```python
from build123d import *

# Parameters (mm, degrees)
SKETCH1_R           = 8.5
SKETCH1_R_2         = 2.5
BOSS_EXTRUDE2_DEPTH = 4.5


with BuildPart() as part:
    # Sketch1 → Boss-Extrude2 (new body)
    # profile 1 of 3: a face of its own
    with BuildSketch(Plane(origin=(0, 0, 0), x_dir=(1, 0, 0), z_dir=(0, 1, 0))):
        with BuildLine():
            Line((0, 8.5), (-120, 8.5))
            ThreePointArc((-120, 8.5), (-113.98959236, 6.01040764), (-111.5, 0))
            ThreePointArc((-111.5, 0), (-113.98959236, -6.01040764), (-120, -8.5))
            Line((-120, -8.5), (0, -8.5))
            ThreePointArc((0, -8.5), (-8.5, 0), (0, 8.5))
        make_face()
    # profile 2 of 3: a face of its own
    with BuildSketch(Plane(origin=(0, 0, 0), x_dir=(1, 0, 0), z_dir=(0, 1, 0))):
        with Locations((-120, 0)):
            Circle(SKETCH1_R)
        with Locations(Location((-120, 0, 0), (0, 0, 270))):
            Circle(SKETCH1_R_2, mode=Mode.SUBTRACT)
    # profile 3 of 3: a face of its own
    with BuildSketch(Plane(origin=(0, 0, 0), x_dir=(1, 0, 0), z_dir=(0, 1, 0))):
        Circle(SKETCH1_R)
        with Locations(Location((0, 0, 0), (0, 0, 270))):
            Circle(SKETCH1_R_2, mode=Mode.SUBTRACT)
    extrude(amount=BOSS_EXTRUDE2_DEPTH)


solid = part.part
```
Part model, mm, in its own coordinate system. Give positions to 0.01 mm unless a question says otherwise; leave off trailing zeros. Order: outer loops, then holes, each group sorted by start corner. A loop starts at its lowest first (then second) coordinate and runs counter-clockwise, first axis right, second up. Notation, with made-up numbers: M -32,-2 L 20,-2 A26 ccw 20,24 Z; hole C 69.25,8 d6. An arc over 180 degrees is marked long. Use a Markdown table: item, result. Add a question column.
(1) Saw through at B-B, the plane y = 3.1. Give the cut face in (x, z).
(2) Saw through at D-D, the plane z = -7. Give the cut face in (x, y), and give its area (3 significant figures).
(3) Mould opens along X. For faces 1 (the face through (-61, 4.5, 0)), 2 (the face through (-128.498, 2.218, -0.187)), 3 (the face through (-117.52, 2.22, -0.33)) say: +X half, -X half, draft (parallel to the pull), parting line (faces both ways), or undercut.
(4) Saw through at C-C, the plane z = 6.5. Give the cut face in (x, y).
(5) Probe line 1 along X through (y, z) = (0.95, 0); line 2 along X through (y, z) = (1.35, 1.5); line 3 along X through (y, z) = (3.9, -3). List the from-to ranges inside material, lowest first. Write a range as [from, to].
(6) Saw through at A-A, the plane z = 0. Give the cut face in (x, y).
Answer key:
| question | item | result |
|---|---|---|
| 1 | outline | M -120,-8.5 L 0,-8.5 A8.5 ccw 0,8.5 L -120,8.5 A8.5 ccw Z; hole C -120,0 d5; hole C 0,0 d5 |
| 2 | outline | M -124.82,0 L 4.82,0 L 4.82,4.5 L -124.82,4.5 Z |
| 2 | area | 583 mm^2 |
| 3 | face 1 | draft |
| 3 | face 2 | -X half |
| 3 | face 3 | undercut |
| 4 | outline | M -125.48,0 L 5.48,0 L 5.48,4.5 L -125.48,4.5 Z |
| 5 | line 1 | [-128.5, -122.5], [-117.5, -2.5], [2.5, 8.5] |
| 5 | line 2 | [-128.37, -122], [-118, -2], [2, 8.37] |
| 5 | line 3 | [-127.95, 7.95] |
| 6 | outline | M -128.5,0 L -122.5,0 L -122.5,4.5 L -128.5,4.5 Z; M -117.5,0 L -2.5,0 L -2.5,4.5 L -117.5,4.5 Z; M 2.5,0 L 8.5,0 L 8.5,4.5 L 2.5,4.5 Z |
